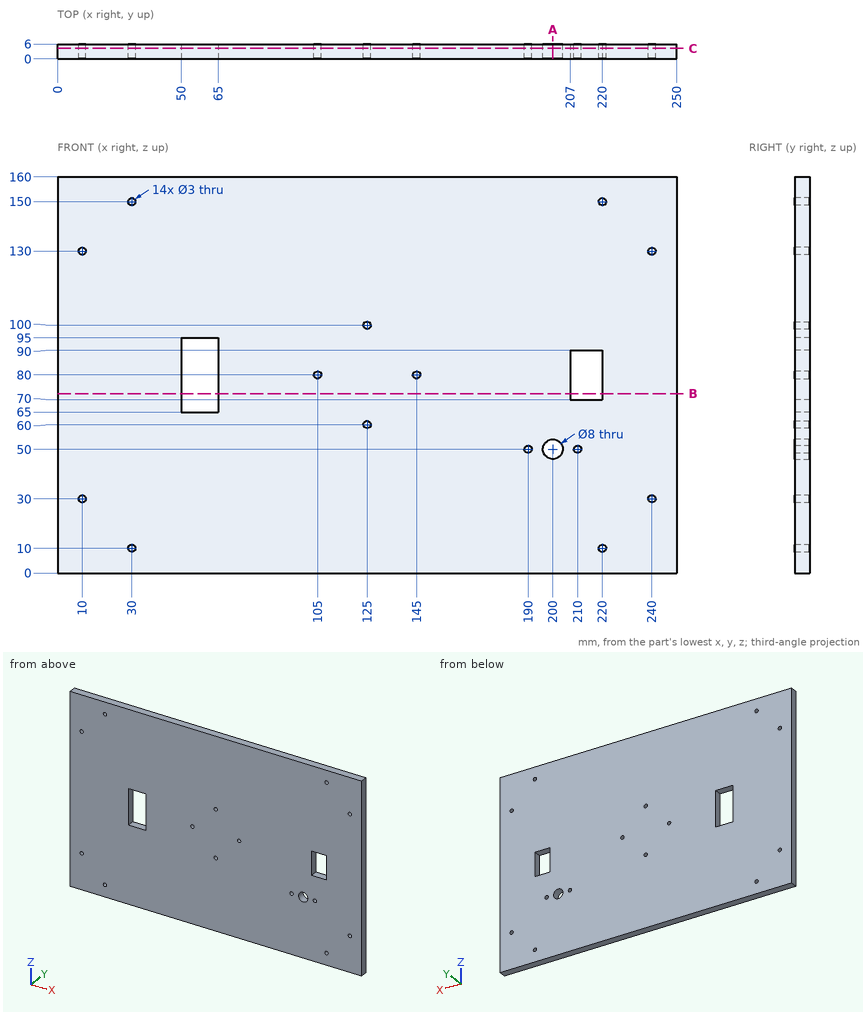
Study the drawing (mm; zero at the part's minimum x, y, z) and answer. Round coordinates to 2 decimals unless told otherwise and drop trailing zeros. Write each loop counter-clockwise with the first axis right and the second up, starting at its lowest first coordinate (ties: lowest second). Pieces come first, ordered by that corner, then holes. Notation, with made-up numbers: (27, 27.25) -> (62, 27.25) arc R27 cw to (62, 46.25) -> close; hole circle Ø1 at (23, -9). An arc over 180 degrees is marked (long way). Write item = value, one per line.
1) Section A-A on x = 200 is taken. Write down the section's boundary in (y, z).
Check values:
outline = (0, 0) -> (6, 0) -> (6, 46) -> (0, 46) -> close; (0, 54) -> (6, 54) -> (6, 160) -> (0, 160) -> close
2) Section C-C on y = 4.2 is taken. Give the number of separate pieces and of enclosed holes in the cut face, plus the area to 3 significant figures.
Check values:
separate_pieces = 1
enclosed_holes = 17
area = 39,100 mm²
3) Given pin 1 (2.5 mm diameter, centred on x = 30, z = 150, fed in from +Y) (3 decimals), flat-ended and moving along its own axis, determine where the tip first touches the part or whether it passes through.
Check values:
pin_1 = through
4) Straight lines are drawn through the part: line 1 along X through (y, z) = (1.9, 50); line 2 along X through (y, z) = (3.75, 10); line 3 along X through (y, z) = (3.3, 80). For each, find the intervals that lie inside material, in ascending order. Write a range as [from, to].
Check values:
line_1 = [0, 188.5], [191.5, 196], [204, 208.5], [211.5, 250]
line_2 = [0, 28.5], [31.5, 218.5], [221.5, 250]
line_3 = [0, 50], [65, 103.5], [106.5, 143.5], [146.5, 207], [220, 250]
5) Section B-B on z = 72.5 is taken. Write down the section's boundary in (x, y), plus the area to 3 significant figures.
Check values:
outline = (0, 0) -> (50, 0) -> (50, 6) -> (0, 6) -> close; (65, 0) -> (207, 0) -> (207, 6) -> (65, 6) -> close; (220, 0) -> (250, 0) -> (250, 6) -> (220, 6) -> close
area = 1,330 mm²
